Part model, mm, in its own coordinate system. A direction names the side the tool comes from. Round coordinates to 2 decimals unless told otherwise and drop trailing zeros. Write each loop counter-clockwise with the first axis right and the second up, starting at its lowest first coordinate (ties: lowest second). Pieces come first, ordered by that corner, then holes. Notation, with made-up numbers: (2.25, -4.5) -> (44.25, -4.5) arc R16 cw to (44.25, 15.5) -> close; hole circle Ø8 at (70.25, 64.5). An arc over 180 degrees is marked (long way). Return JSON: item names as keys, results as strings. Group by question number.
(1) Mould opens along Y. For faces 1 (the cylindrical face through (-0.69, -3.1, -26.4)), 2 (the flat face through (1.4, -2.1, 45)), 3 (the cylindrical face through (-0.5, -2.23, -0.63)) say: +Y half, -Y half, draft (parallel to the pull), parting line (faces both ways), or undercut.
(2) Saw through at A-A (x = 0). List the corners of the cut face in (y, z) (3 decimals).
(3) Drill centre lines: L1, parallel to Y at x = 0, z = 20.5 (3 decimals); L2, parallel to X at y = 1.75, z = -2; L3, parallel to X at y = 1.25, z = -39.5. Where is each one in solid material? Low to high. Write a range as from..to.
(4) Saw through at D-D (y = 5.5). List the corners of the cut face in (x, z).
(5) Drop flat-ended pins along their axis: pin 1 Ø8 at (x, z) = (1.5, 23) entering from +Y (3 decimals); pin 2 Ø4 at (x, z) = (-1, 3) entering from -Y; pin 3 Ø1.5 at (x, z) = (-4, 28) entering from -Y; pin 4 Ø1 at (x, z) = (1.5, 3.5) entering from -Y. Give the stop position or say it passes through.
(6) Tool access for faces 4 (the cylindrical face through (-0.69, -3.1, 25.87)), 5 (the flat face through (1.4, -2.1, -45)): list every direction of +Z, -Z, +X, -X, +Y, -Y with a clear straight run to the whole face (end or side of a thin tool).
(7) Saw through at C-C (z = -32). List the corners of the cut face in (x, y) (3 decimals).
from build123d import *

# Parameters (mm, degrees)
CUT_EXTRUDE1_DEPTH       = 14.743823158
CUT_EXTRUDE1_DEPTH_BACK  = 14.743823158
SKETCH4_R                = 3.175
BOSS_EXTRUDE1_DEPTH      = 45
BOSS_EXTRUDE1_DEPTH_BACK = 45
SKETCH5_R                = 3.175
SKETCH5_R_2              = 2.286


with BuildPart() as part:
    # Sketch3 → Revolve3 (revolve)
    with BuildSketch(Plane(origin=(0, 0, 0), x_dir=(1, 0, 0), z_dir=(0, 1, 0))):
        with BuildLine():
            Line((0, -7.935), (0, 7.935))
            ThreePointArc((0, 7.935), (-7.935, 0), (0, -7.935))
        make_face()
    revolve(axis=Axis((0, 0, -12.438098035), (0, 0, 1)))

    # Sketch4 → Cut-Extrude1 (cut, two sides: drawn at the far end of the back side and taken through both)
    with BuildSketch(Plane.XY.offset(-CUT_EXTRUDE1_DEPTH_BACK)):
        Circle(SKETCH4_R)
    extrude(amount=CUT_EXTRUDE1_DEPTH + CUT_EXTRUDE1_DEPTH_BACK, mode=Mode.SUBTRACT)

    # Sketch5 → Boss-Extrude1 (add, two sides: drawn at the far end of the back side and taken through both)
    with BuildSketch(Plane.XY.offset(-BOSS_EXTRUDE1_DEPTH_BACK)):
        Circle(SKETCH5_R)
        Circle(SKETCH5_R_2, mode=Mode.SUBTRACT)
    extrude(amount=BOSS_EXTRUDE1_DEPTH + BOSS_EXTRUDE1_DEPTH_BACK)


solid = part.part
Computed values:
{
 "1": {"face 1": "parting line", "face 2": "draft", "face 3": "undercut"},
 "2": {"outline": "(-3.175, -45) -> (-2.286, -45) -> (-2.286, 45) -> (-3.175, 45) -> (-3.175, 7.272) arc R7.935 ccw to (-3.175, -7.272) -> close; (2.286, -45) -> (3.175, -45) -> (3.175, -7.272) arc R7.935 ccw to (3.175, 7.272) -> (3.175, 45) -> (2.286, 45) -> close"},
 "3": {"L1": "-3.175..-2.286, 2.286..3.175", "L2": "-7.48..-1.47, 1.47..7.48", "L3": "-2.92..-1.91, 1.91..2.92"},
 "4": {"outline": "circle Ø11.44 at (0, 0)"},
 "5": {"pin 1": "y = 3.175", "pin 2": "y = -7.85", "pin 3": "through", "pin 4": "y = -7.21"},
 "6": {"face 4": "+Z", "face 5": "-Z, +X, -X, +Y, -Y"},
 "7": {"outline": "circle Ø6.35 at (0, 0); hole circle Ø4.572 at (0, 0)"}
}
